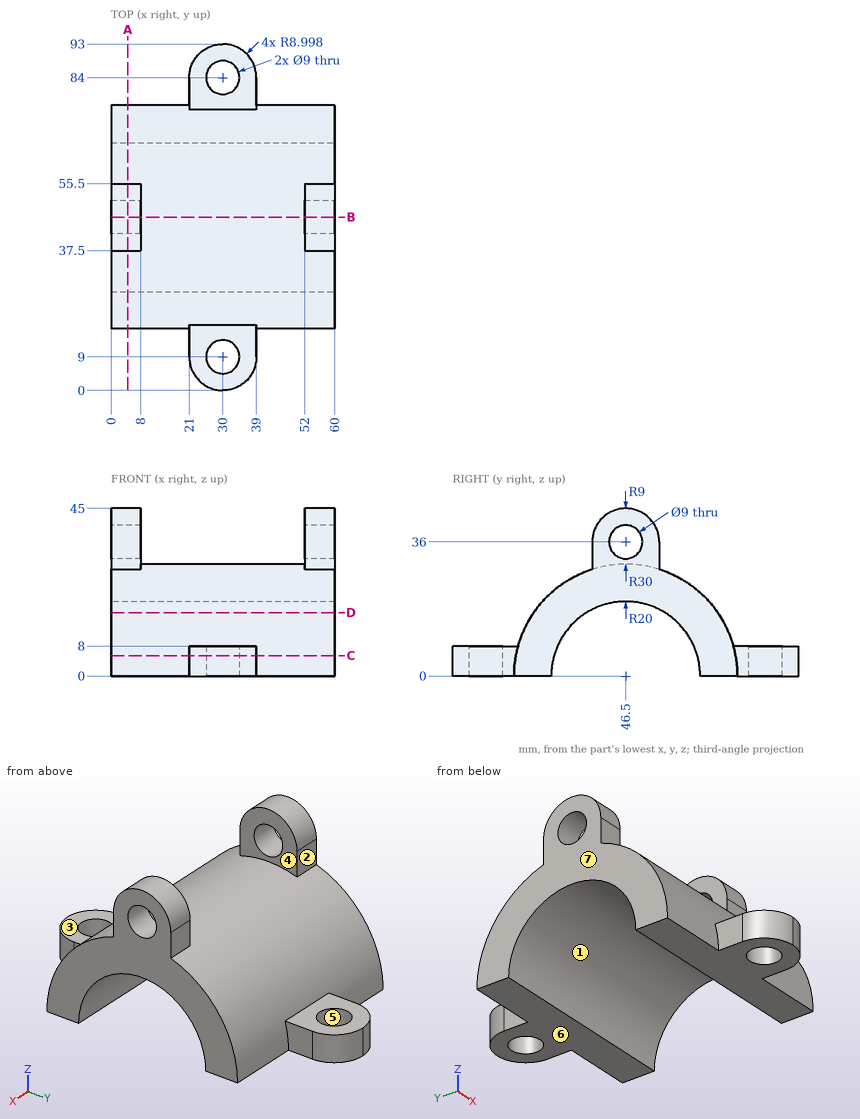
Design review of the part shown in the three views and the two pictorial views. Dimensions are in mm from the part's minimum x, y and z. A direction names the side the tool comes from. Round coordinates to 2 decimals unless told otherwise and drop trailing zeros. Order: outer loops, then holes, each group sorted by start corner. A loop starts at its lowest first (then second) coordinate and runs counter-clockwise, first axis right, second up.
Q1. We need section D-D, the plane z = 17. Give the boundary of the cut face in (x, y), plus the area to 3 significant figures.
Findings below:
outline: (0, 21.78) - (60, 21.78) - (60, 35.96) - (0, 35.96) - close; (0, 57.04) - (60, 57.04) - (60, 71.22) - (0, 71.22) - close
area: 1,700 mm2
Q2. We need section B-B, the plane y = 46.5. Give the boundary of the cut face in (x, z).
Findings below:
outline: (0, 20) - (60, 20) - (60, 31.5) - (52, 31.5) - (52, 30) - (8, 30) - (8, 31.5) - (0, 31.5) - close; (0, 40.5) - (8, 40.5) - (8, 45) - (0, 45) - close; (52, 40.5) - (60, 40.5) - (60, 45) - (52, 45) - close
Q3. We need section C-C, the plane z = 5.5. State how many separate pieces and enclosed holes the cut face has, plus the area to 3 significant figures.
Findings below:
separate pieces: 2
enclosed holes: 2
area: 1,650 mm2
Q4. Insertion check: P1, Ø18, axis at y = 46, z = 38, coming from the -X side; P2, Ø14.5, axis at x = 30, y = 84, coming from the +Z side; P3, Ø8, axis at y = 78.5, z = 14, coming from the +X side; P4, Ø3.5, axis at x = 55, z = 33, coming from the +Y side. Each pin has a flat end and moves straight along its axis. Give the tip position at first contact, or say it passes through.
Findings below:
P1: stops at x = 0
P2: stops at z = 8
P3: passes through
P4: stops at y = 55.5
Q5. We need section A-A, the plane x = 4.5. Give the boundary of the cut face in (y, z), plus the area to 3 significant figures.
Findings below:
outline: (16.5, 0) - (26.5, 0) arc R20 cw to (66.5, 0) - (76.5, 0) arc R30 ccw to (55.5, 28.62) - (55.5, 36) arc R9 ccw to (37.5, 36) - (37.5, 28.62) arc R30 ccw to start; hole circle Ø9 at (46.5, 36)
area: 965 mm2
Q6. Mouldability with a two-part tool opening along X and no side actions: class the marked faces 4, 5, 6 and 7 as pulls with the +X half, pulls with the -X half, needs draft (parallel to the pull), parting line crosses it, or undercut.
Findings below:
face 4: undercut
face 5: undercut
face 6: needs draft
face 7: pulls with the -X half
Q7. Wall thickness on line 1 (Z direction, x = 56, y = 46.5); line 2 (X direction, y = 9, z = 1); line 3 (Y direction, x = 30, z = 6.25): over which ranges is each line inside the solid? List them lowest first.
Findings below:
line 1: z = 20 to 31.5, 40.5 to 45
line 2: x = 21 to 25.5, 34.5 to 39
line 3: y = 0 to 4.5, 13.5 to 27.5, 65.5 to 79.5, 88.5 to 93
Q8. Machinability: for the marked faces 1, 2 and 3, which of the approach directions +Z, -Z, +X, -X, +Y, -Y give a long, thin tool a straight path to every point of the face, cutting with its end or side? Answer none if there is none.
Findings below:
face 1: -Z, +X, -X
face 2: +Z, +X, -X, +Y
face 3: +Z, +X, -X, -Y
